Model file for the job. Use its own axes, mm. A direction names the side the tool comes from. Give positions to 0.01 mm unless a question says otherwise; leave off trailing zeros. Write each loop counter-clockwise with the first axis right and the second up, starting at its lowest first coordinate (ties: lowest second). Pieces come first, ordered by that corner, then holes.
```python
from build123d import *

# Parameters (mm, degrees)
SKETCH1_W             = 140
SKETCH1_H             = 40
BOSS_EXTRUDE1_DEPTH   = 15
BOSS_EXTRUDE2_DEPTH   = 1.5
BOSS_EXTRUDE3_DEPTH   = 1.5
BOSS_EXTRUDE4_DEPTH   = 1.5
FILLET2_R             = 0.25
MIRROR10_COPY_1_DEPTH = 1.5
MIRROR11_COPY_1_DEPTH = 1.5
MIRROR11_COPY_2_DEPTH = 1.5
MIRROR11_COPY_3_DEPTH = 1.5
MIRROR11_COPY_4_DEPTH = 1.5
SKETCH2_W             = 129
SKETCH2_H             = 28
BOSS_EXTRUDE5_DEPTH   = 7.5
SKETCH8_W             = 127
SKETCH8_H             = 26
CUT_EXTRUDE1_DEPTH    = 10
CUT_EXTRUDE2_DEPTH    = 41.5
CUT_EXTRUDE3_DEPTH    = 41.5
FILLET3_R             = 0.25
FILLET4_R             = 0.25


with BuildPart() as part:
    # Sketch1 → Boss-Extrude1 (new body)
    with BuildSketch(Plane(origin=(0, 0, 0), x_dir=(1, 0, 0), z_dir=(0, 1, 0))):
        Rectangle(SKETCH1_W, SKETCH1_H)
    extrude(amount=BOSS_EXTRUDE1_DEPTH)

    # Sketch3 → Boss-Extrude2 (add, symmetric)
    with BuildSketch(Plane.XY):
        Polygon((-65.5, 15), (-65.5, 21.5), (-69.845299462, 21.5), (-71, 19.5), (-68.5, 19.5), (-68.5, 15), align=None)
    boss_extrude2 = extrude(amount=BOSS_EXTRUDE2_DEPTH, both=True)

    # Sketch6 → Boss-Extrude3 (add)
    with BuildSketch(Plane(origin=(0, 0, 0), x_dir=(0, 0, -1), z_dir=(1, 0, 0))):
        Polygon((-15, 15), (-15, 21.5), (-19.345299462, 21.5), (-20.5, 19.5), (-18, 19.5), (-18, 15), align=None)
    boss_extrude3 = extrude(amount=-BOSS_EXTRUDE3_DEPTH)

    # Sketch7 → Boss-Extrude4 (add, symmetric)
    with BuildSketch(Plane(origin=(-35, 0, 0), x_dir=(0, 0, -1), z_dir=(1, 0, 0))):
        Polygon((-15, 15), (-15, 21.5), (-19.345299462, 21.5), (-20.5, 19.5), (-18, 19.5), (-18, 15), align=None)
    boss_extrude4 = extrude(amount=BOSS_EXTRUDE4_DEPTH, both=True)

    # Fillet2
    fillet2_edges = [part.edges().sort_by_distance(p)[0] for p in [
        (-71, 19.5, 0),
    ]]
    fillet(fillet2_edges, radius=FILLET2_R)

    # Mirror9: Boss-Extrude3 across plane
    add(boss_extrude3.mirror(Plane(origin=(0, 0, 0), x_dir=(0, 0, 1), z_dir=(1, 0, 0))))

    # Mirror10: Boss-Extrude4, Boss-Extrude3 across plane
    add(boss_extrude4.mirror(Plane.XY))
    add(boss_extrude3.mirror(Plane.XY))

    # Mirror10 copy 1 sketch → Mirror10 copy 1 (add)
    with BuildSketch(Plane.ZY):
        Polygon((-15, 15), (-15, 21.5), (-19.345299462, 21.5), (-20.5, 19.5), (-18, 19.5), (-18, 15), align=None)
    extrude(amount=-MIRROR10_COPY_1_DEPTH)

    # Mirror11: Boss-Extrude2, Boss-Extrude4 across plane
    add(boss_extrude2.mirror(Plane(origin=(0, 0, 0), x_dir=(0, 0, 1), z_dir=(1, 0, 0))))
    add(boss_extrude4.mirror(Plane(origin=(0, 0, 0), x_dir=(0, 0, 1), z_dir=(1, 0, 0))))

    # Mirror11 copy 1 sketch → Mirror11 copy 1 (add, symmetric)
    with BuildSketch(Plane.ZY.offset(-35)):
        Polygon((-15, 15), (-15, 21.5), (-19.345299462, 21.5), (-20.5, 19.5), (-18, 19.5), (-18, 15), align=None)
    extrude(amount=MIRROR11_COPY_1_DEPTH, both=True)

    # Mirror11 copy 2 sketch → Mirror11 copy 2 (add)
    with BuildSketch(Plane.ZY):
        Polygon((-15, 15), (-15, 21.5), (-19.345299462, 21.5), (-20.5, 19.5), (-18, 19.5), (-18, 15), align=None)
    extrude(amount=-MIRROR11_COPY_2_DEPTH)

    # Mirror11 copy 3 sketch → Mirror11 copy 3 (add)
    with BuildSketch(Plane(origin=(0, 0, 0), x_dir=(0, 0, 1), z_dir=(1, 0, 0))):
        Polygon((-15, -15), (-15, -21.5), (-19.345299462, -21.5), (-20.5, -19.5), (-18, -19.5), (-18, -15), align=None)
    extrude(amount=-MIRROR11_COPY_3_DEPTH)

    # Mirror11 copy 4 sketch → Mirror11 copy 4 (add)
    with BuildSketch(Plane(origin=(0, 0, 0), x_dir=(0, 0, -1), z_dir=(-1, 0, 0))):
        Polygon((-15, -15), (-15, -21.5), (-19.345299462, -21.5), (-20.5, -19.5), (-18, -19.5), (-18, -15), align=None)
    extrude(amount=-MIRROR11_COPY_4_DEPTH)

    # Sketch2 → Boss-Extrude5 (add)
    with BuildSketch(Plane(origin=(0, 15, 0), x_dir=(1, 0, 0), z_dir=(0, 1, 0))):
        Rectangle(SKETCH2_W, SKETCH2_H)
    extrude(amount=BOSS_EXTRUDE5_DEPTH)

    # Sketch8 → Cut-Extrude1 (cut)
    with BuildSketch(Plane(origin=(0, 22.5, 0), x_dir=(1, 0, 0), z_dir=(0, 1, 0))):
        Rectangle(SKETCH8_W, SKETCH8_H)
    extrude(amount=-CUT_EXTRUDE1_DEPTH, mode=Mode.SUBTRACT)

    # Sketch9 → Cut-Extrude2 (cut, through all)
    with BuildSketch(Plane.XY.offset(20)):
        with BuildLine():
            Line((-4, 7), (4, 7))
            ThreePointArc((4, 7), (5.5, 5.5), (4, 4))
            Line((4, 4), (-4, 4))
            ThreePointArc((-4, 4), (-5.5, 5.5), (-4, 7))
        make_face()
    extrude(amount=-CUT_EXTRUDE2_DEPTH, mode=Mode.SUBTRACT)

    # Sketch10 → Cut-Extrude3 (cut, through all)
    with BuildSketch(Plane.XY.offset(20)):
        with BuildLine():
            Line((-39, 7), (-31, 7))
            ThreePointArc((-31, 7), (-29.5, 5.5), (-31, 4))
            Line((-31, 4), (-39, 4))
            ThreePointArc((-39, 4), (-40.5, 5.5), (-39, 7))
        make_face()
    cut_extrude3 = extrude(amount=-CUT_EXTRUDE3_DEPTH, mode=Mode.SUBTRACT)

    # Mirror12: Cut-Extrude3 across plane
    add(cut_extrude3.mirror(Plane(origin=(0, 0, 0), x_dir=(0, 0, 1), z_dir=(1, 0, 0))), mode=Mode.SUBTRACT)

    # Fillet3
    fillet3_edges = [part.edges().sort_by_distance(p)[0] for p in [
        (0, 19.5, -20.5),
        (71, 19.5, 0),
        (35, 19.5, -20.5),
        (35, 19.5, 20.5),
        (0, 19.5, 20.5),
        (-35, 19.5, 20.5),
        (-35, 19.5, -20.5),
    ]]
    fillet(fillet3_edges, radius=FILLET3_R)

    # Fillet4
    fillet4_edges = [part.edges().sort_by_distance(p)[0] for p in [
        (0, 15, -15),
        (0, 15, -18),
        (65.5, 15, 0),
        (35, 15, -15),
        (35, 15, -18),
        (-65.5, 15, 0),
        (-68.5, 15, 0),
        (35, 15, 18),
        (35, 15, 15),
        (0, 15, 15),
        (0, 15, 18),
        (-35, 15, 15),
        (-35, 15, 18),
        (-35, 15, -18),
        (-35, 15, -15),
    ]]
    fillet(fillet4_edges, radius=FILLET4_R)


solid = part.part
```
1. Pull direction Z, two halves, no side cores. Call faces 5 (the flat face through (-1, 7.4, -20)), 6 (the flat face through (-1, 18, -13)), 7 (the flat face through (35, 18, -15)), 8 (the flat face through (-33.5, 19, 17)): +Z half, -Z half, draft (parallel to the pull), parting line (faces both ways), or undercut.
Calculated:
face 5: -Z half
face 6: undercut
face 7: undercut
face 8: draft
2. Slice it at A-A, the plane y = 5.5. Write the cut outline in (x, z).
Calculated:
outline: (-70, -20) - (-40.5, -20) - (-40.5, 20) - (-70, 20) - close; (-29.5, -20) - (-5.5, -20) - (-5.5, 20) - (-29.5, 20) - close; (5.5, -20) - (29.5, -20) - (29.5, 20) - (5.5, 20) - close; (40.5, -20) - (70, -20) - (70, 20) - (40.5, 20) - close
3. Slice it at B-B, the plane z = 6. Write the cut outline in (x, y).
Calculated:
outline: (-70, 0) - (70, 0) - (70, 15) - (64.5, 15) - (64.5, 22.5) - (63.5, 22.5) - (63.5, 12.5) - (-63.5, 12.5) - (-63.5, 22.5) - (-64.5, 22.5) - (-64.5, 15) - (-70, 15) - close; hole (-39, 4) - (-31, 4) arc R1.5 ccw to (-31, 7) - (-39, 7) arc R1.5 ccw to start; hole (-4, 4) - (4, 4) arc R1.5 ccw to (4, 7) - (-4, 7) arc R1.5 ccw to start; hole (31, 4) - (39, 4) arc R1.5 ccw to (39, 7) - (31, 7) arc R1.5 ccw to start
4. Slice it at C-C, the plane y = 16.5. State how many separate pieces and enclosed holes the cut face has, and give its area (3 significant figures).
Calculated:
separate pieces: 9
enclosed holes: 1
area: 382 mm2
5. Pin check, flat tips, straight feed: P1, Ø6, axis at x = -20.5, z = -5, coming from the +Y side; P2, Ø6, axis at x = 52, y = 17, coming from the -Z side; P3, Ø5, axis at y = 8.5, z = 14.5, coming from the -X side. Stop position of each tip, or through.
Calculated:
P1: stops at y = 12.5
P2: stops at z = -20
P3: stops at x = -70
6. Which spindle directions (+Z, -Z, +X, -X, +Y, -Y) get a long thin tool onto all of the face, cutting with end or side? Do faces 1 (the flat face through (0, 17, 18)), 2 (the flat face through (35, 18, 15)), 3 (the flat face through (35, 17, -18)), 4 (the cylindrical face through (-40.5, 5.5, 0.3)). Say none if no direction does.
Calculated:
face 1: +Z, +X, -X
face 2: +X, -X, +Y
face 3: -Z, +X, -X
face 4: +Z, -Z
7. Probe probe 1 along X at (y, z) = (20, 19); probe 2 along Z at (x, y) = (-50, 13.75); probe 3 along Z at (x, y) = (57, 16). List the from-to ranges inside material, lowest first.
Calculated:
probe 1: x = -36.5 to -33.5, -1.5 to 1.5, 33.5 to 36.5
probe 2: z = -20 to -13, 13 to 20
probe 3: z = -14 to -13, 13 to 14
8. Slice it at D-D, the plane x = -23. Write the cut outline in (y, z).
Calculated:
outline: (0, -20) - (15, -20) - (15, -14) - (22.5, -14) - (22.5, -13) - (12.5, -13) - (12.5, 13) - (22.5, 13) - (22.5, 14) - (15, 14) - (15, 20) - (0, 20) - close
